Build history of the part. All positions in model axes, mm. A direction names the side the tool comes from. Round coordinates to 2 decimals unless told otherwise and drop trailing zeros. Write each loop counter-clockwise with the first axis right and the second up, starting at its lowest first coordinate (ties: lowest second). Pieces come first, ordered by that corner, then holes. Notation, with made-up numbers: M 42.25,57.5 L 89.25,57.5 A25 cw 89.25,83.5 Z; hole C 57,6 d2. An arc over 180 degrees is marked long. Use a Markdown table: item, result.
from build123d import *

# Parameters (mm, degrees)
F0_R          = 15
F1_DEPTH      = 120
F1_DEPTH_BACK = 50
F3_START      = 2
F3_DEPTH      = 23
F4_DEPTH      = 25


with BuildPart() as f1:
    # F0 (on Top) → F1 (new body, two sides)
    with BuildSketch(Plane.XY) as f1_sk:
        Circle(F0_R)
    extrude(amount=F1_DEPTH)
    extrude(f1_sk.sketch, amount=-F1_DEPTH_BACK)

    # F2 (on Front) → F3 (cut)
    with BuildSketch(Plane.XZ.offset(F3_START)):
        Polygon((-17.8860742599, 120), (-17, 105), (-17, 84.1139257401), (-2, 100), (-2, 105), align=None)
        Polygon((-17, 70), (-17, 84.1139257401), (-17.8860742599, 83.1755096406), align=None)
        Polygon((2, 100), (17, 84.1139257401), (17, 105), (17.8860742599, 120), (2, 105), align=None)
        Polygon((17, 70), (17.8860742599, 83.1755096406), (17, 84.1139257401), align=None)
    extrude(amount=F3_DEPTH, mode=Mode.SUBTRACT)

    # F2 (on Front) → F4 (cut)
    with BuildSketch(Plane.XZ):
        Polygon((-17.8860742599, 120), (-17, 105), (-17, 84.1139257401), (-2, 100), (-2, 105), align=None)
        Polygon((-17, 70), (-17, 84.1139257401), (-17.8860742599, 83.1755096406), align=None)
        Polygon((2, 100), (17, 84.1139257401), (17, 105), (17.8860742599, 120), (2, 105), align=None)
        Polygon((17, 70), (17.8860742599, 83.1755096406), (17, 84.1139257401), align=None)
    extrude(amount=-F4_DEPTH, mode=Mode.SUBTRACT)

    # F5 (on Front) → F6 (revolve, cut)
    with BuildSketch(Plane.XZ):
        Polygon((0, 123.1170922147), (-15.8692053304, 123.1170922147), (-1, 110.1170922147), (-1, 65.1170922147), (-13.300107735, 50.4583946322), (-13.300107735, -8.0997264013), (0, -8.0997264013), (0, 65.1170922147), (0, 110.1170922147), align=None)
    revolve(axis=Axis((0, 0, 116.6170922147), (0, 0, -1)), mode=Mode.SUBTRACT)


solid = f1.part
Q1. Cut at B-B on z = 94. Give the cut face in (x, y).
Response values:
| item | result |
|---|---|
| outline | M -15,0 A15 ccw -14.87,-2 L -7.67,-2 L -7.67,-12.89 A15 ccw 7.67,-12.89 L 7.67,-2 L 14.87,-2 A15 ccw 15,0 L 7.67,0 L 7.67,12.89 A15 ccw -7.67,12.89 L -7.67,0 Z; hole C 0,0 d2 |
Q2. Cut at C-C on z = -33. Give the cut face in (x, y).
Response values:
| item | result |
|---|---|
| outline | C 0,0 d30 |
Q3. Cut at D-D on z = 39. Give the cut face in (x, y).
Response values:
| item | result |
|---|---|
| outline | C 0,0 d30; hole C 0,0 d26.6 |
Q4. Drill centre lines: L1, parallel to Y at x = 0, z = 80; L2, parallel to Y at x = 0, z = 4; L3, parallel to Z at x = 12.25, y = 2.25. Where is each one in solid material? Low to high.
Response values:
| item | result |
|---|---|
| L1 | y = -15 to -1, 1 to 15 |
| L2 | y = -15 to -13.3, 13.3 to 15 |
| L3 | z = -50 to -8.1, 51.47 to 89.14, 114.68 to 120 |
Q5. Two-plate mould, pull along Y, no slides. Class faces 6 (the cylindrical face through (14.307, 4.506, 36.19)), 7 (the flat face through (2, -8, 103)), 8 (the cylindrical face through (2.883, -12.984, 20.769)): +Y half, -Y half, draft (parallel to the pull), parting line (faces both ways), or undercut.
Response values:
| item | result |
|---|---|
| face 6 | parting line |
| face 7 | draft |
| face 8 | undercut |
Q6. Drop flat-ended pins along their axis: P1, Ø6.5, axis at x = 6.5, z = 96, coming from the -Y side; P2, Ø2, axis at x = -11, z = 88.5, coming from the +Y side; P3, Ø1.5, axis at y = 6.5, z = 101.5, coming from the +X side. Give the stop position or say it passes through.
Response values:
| item | result |
|---|---|
| P1 | stops at y = -14.64 |
| P2 | stops at y = 11.18 |
| P3 | stops at x = 2 |
Q7. Which spindle directions (+Z, -Z, +X, -X, +Y, -Y) get a long thin tool onto all of the face, cutting with end or side? Do faces 1 (the flat face through (0, 0, -8.1)), 2 (the flat face through (-6.913, -6.913, 109.639)), 3 (the flat face through (7.15, 5.68, 109.86)), 4 (the flat face through (10, -2, 102)), 5 (the flat face through (-6.965, 5.677, 109.688)). Say none if no direction does.
Response values:
| item | result |
|---|---|
| face 1 | none |
| face 2 | -X, -Y |
| face 3 | +X, +Y |
| face 4 | +X, -Y |
| face 5 | -X, +Y |
Q8. Cut at A-A on z = 67.5. Give the cut face in (x, y), and give its area (3 significant figures).
Response values:
| item | result |
|---|---|
| outline | C 0,0 d30; hole C 0,0 d2 |
| area | 704 mm2 |
